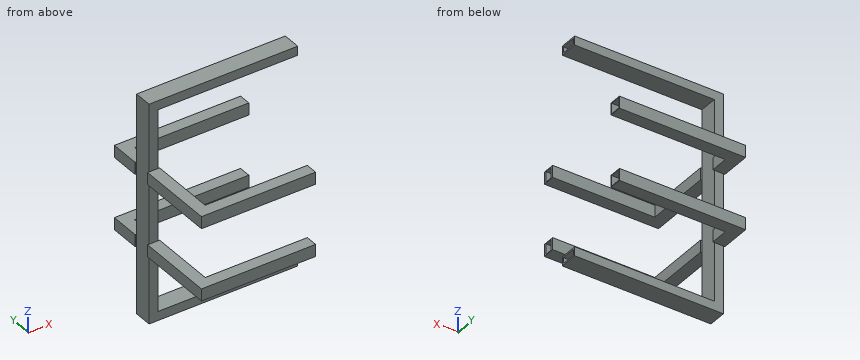
Autodesk Inventor part; units mm, degrees
ref_plane "Work Plane2" through (304.8, 0, 0) normal (1, 0, 0) x (0, 1, 0)
ref_plane "Work Plane3" through (0, 0, 50.8) normal (0, 0, 1) x (1, 0, 0)
ref_plane "Work Plane5" through (0, 0, 76.2) normal (0, 0, 1) x (1, 0, 0)
sketch "Sketch10" plane through (0, 0, 0) normal (0, 1, 0) x (-1, 0, 0)
  line L0 (0, 0) -> (0, 222.25)
  line L1 (0, 222.25) -> (-304.8, 222.25)
  line L2 (0, 0) -> (-304.8, 0) construction
  line L3 (0, 0) -> (0, -222.25)
  line L4 (0, -222.25) -> (-304.8, -222.25)
  dimension "d31" = 222.25
  dimension "d32" = 304.8
ref_plane "Work Plane2" through (304.8, 0, 0) normal (1, 0, 0) x (0, 1, 0)
sketch "Sketch11" plane through (304.8, 0, 0) normal (1, 0, 0) x (0, 1, 0)
  line L0 (-19.05, 231.775) -> (-19.05, 212.725)
  line L1 (-19.05, 212.725) -> (19.05, 212.725)
  line L2 (19.05, 212.725) -> (19.05, 231.775)
  line L3 (19.05, 231.775) -> (-19.05, 231.775)
  line L4 (-19.05, 231.775) -> (19.05, 212.725) construction
  line L5 (-19.05, 212.725) -> (19.05, 231.775) construction
  line L6 (-15.875, 228.6) -> (-15.875, 215.9)
  line L7 (-15.875, 215.9) -> (15.875, 215.9)
  line L8 (15.875, 215.9) -> (15.875, 228.6)
  line L9 (15.875, 228.6) -> (-15.875, 228.6)
  line L10 (-15.875, 228.6) -> (15.875, 215.9) construction
  line L11 (-15.875, 215.9) -> (15.875, 228.6) construction
  point P0 (0, 0)
  point P1 (0, 222.25)
  dimension "d34" = 222.25
  dimension "d35" = 19.05
  dimension "d36" = 38.1
  dimension "d37" = 3.175
  dimension "d38" = 3.175
sweep "Sweep5" add profiles "Sketch11" path "Sketch10"
sketch "Sketch12" plane through (304.8, 19.05, 231.775) normal (0, 1, 0) x (1, 0, 0)
  line L0 (-304.8, 231.775) -> (-304.8, 0) construction
  line L1 (0, 0) -> (-314.325, 0) construction
  line L2 (-317.5, 142.875) -> (-292.1, 142.875)
  line L3 (-292.1, 142.875) -> (-292.1, 168.275)
  line L4 (-292.1, 168.275) -> (-317.5, 168.275)
  line L5 (-317.5, 168.275) -> (-317.5, 142.875)
  line L6 (-317.5, 142.875) -> (-292.1, 168.275) construction
  line L7 (-292.1, 142.875) -> (-317.5, 168.275) construction
  line L8 (-298.45, 15.875) -> (-298.45, 447.675)
  line L9 (-315.9125, 144.4625) -> (-293.6875, 144.4625)
  line L10 (-293.6875, 144.4625) -> (-293.6875, 166.6875)
  line L11 (-293.6875, 166.6875) -> (-315.9125, 166.6875)
  line L12 (-315.9125, 166.6875) -> (-315.9125, 144.4625)
  line L13 (-315.9125, 144.4625) -> (-293.6875, 166.6875) construction
  line L14 (-293.6875, 144.4625) -> (-315.9125, 166.6875) construction
  point P0 (-304.8, 155.575)
  dimension "d41" = 25.4
  dimension "d42" = 25.4
  dimension "d43" = 76.2
  dimension "d44" = 1.5875
  dimension "d45" = 1.5875
ref_plane "Work Plane3" through (0, 0, 50.8) normal (0, 0, 1) x (1, 0, 0)
sketch "Sketch13" plane through (0, 0, 50.8) normal (0, 0, 1) x (1, 0, 0)
  line L0 (304.8, 19.05) -> (-9.525, 19.05)
  line L1 (0, 19.05) -> (0, 69.85)
  line L2 (0, 69.85) -> (254, 69.85)
  point P0 (0, 0)
  dimension "d47" = 254
  dimension "d48" = 50.8
sweep "Sweep6" add profiles "Sketch12" path "Sketch13" path curves L1 L2 contours L5 L4 L8 L11 L12 L9 L2 | L8 L9 L10 L11 L4 L3 L2
mirror "Mirror2" about plane through (0, 0, 0) normal (0, 0, 1) of "Sweep6"
sketch "Sketch14" plane through (304.8, -19.05, 212.725) normal (0, -1, 0) x (1, 0, 0)
  line L0 (-304.8, -212.725) -> (-304.8, 15.875) construction
  line L1 (0, 15.875) -> (-311.15, 15.875) construction
  line L2 (-317.5, -123.825) -> (-317.5, -149.225)
  line L3 (-317.5, -149.225) -> (-292.1, -149.225)
  line L4 (-292.1, -149.225) -> (-292.1, -123.825)
  line L5 (-292.1, -123.825) -> (-317.5, -123.825)
  line L6 (-317.5, -123.825) -> (-292.1, -149.225) construction
  line L7 (-317.5, -149.225) -> (-292.1, -123.825) construction
  line L8 (-312.7375, -125.4125) -> (-312.7375, -147.6375)
  line L9 (-312.7375, -147.6375) -> (-296.8625, -147.6375)
  line L10 (-296.8625, -147.6375) -> (-296.8625, -125.4125)
  line L11 (-296.8625, -125.4125) -> (-312.7375, -125.4125)
  line L12 (-312.7375, -125.4125) -> (-296.8625, -147.6375) construction
  line L13 (-312.7375, -147.6375) -> (-296.8625, -125.4125) construction
  line L14 (-314.325, 19.05) -> (-314.325, -444.5)
  point P0 (-304.8, -136.525)
  dimension "d52" = 76.2
  dimension "d53" = 25.4
  dimension "d54" = 25.4
  dimension "d55" = 1.5875
  dimension "d56" = 1.5875
ref_plane "Work Plane5" through (0, 0, 76.2) normal (0, 0, 1) x (1, 0, 0)
sketch "Sketch15" plane through (0, 0, 76.2) normal (0, 0, 1) x (1, 0, 0)
  line L0 (-9.525, -19.05) -> (304.8, -19.05)
  line L1 (0, -19.05) -> (0, -171.45)
  line L2 (0, -171.45) -> (228.6, -171.45)
  point P0 (0, 0)
  dimension "d58" = 228.6
  dimension "d59" = 152.4
sweep "Sweep7" add profiles "Sketch14" path "Sketch15" path curves L1 L2
mirror "Mirror5" about plane through (0, 0, 0) normal (0, 0, 1) of "Sweep7"
ref_plane "Work Plane6" through (152.4, 0, 0) normal (1, 0, 0) x (0, 1, 0)
equation "\"d31\" = halfOfWidth"
equation "\"d32\" = length"
equation "\"d35\" = largeTubingWidth"
equation "\"d36\" = largeTubingHeight"
equation "\"d37\" = largeTubeThickness"
equation "\"d38\" = largeTubeThickness"
equation "\"d41\" = smallSupportTubeWidth"
equation "\"d42\" = smallSupportTubeWidth"
equation "\"d44\" = smallSupportTubeThickness"
equation "\"d45\" = smallSupportTubeThickness"
equation "\"d47\" = topSupportTubeExtension"
equation "\"d48\" = smallSupportTubeLength"
equation "\"d53\" = smallSupportTubeWidth"
equation "\"d54\" = smallSupportTubeHeight"
equation "\"d55\" = smallSupportTubeThickness"
equation "\"d56\" = smallSupportTubeThickness"
equation "\"d58\" = bottomSupportTubeExtension"
equation "\"halfOfWidth\" = 0.5 * width"
equation "\"length\" = 304.8"
equation "\"height\" = 241.3"
equation "\"largeTubingWidth\" = 19.05"
equation "\"largeTubingHeight\" = 38.1"
equation "\"largeTubeThickness\" = 3.175"
equation "\"d33\" = length"
equation "\"width\" = 444.5"
equation "\"smallSupportTubeWidth\" = 25.4"
equation "\"smallSupportTubeHeight\" = 25.4"
equation "\"smallSupportTubeThickness\" = 1.5875"
equation "\"distaceToMiddleSmallSupportTube\" = 76.2"
equation "\"smallSupportTubeLength\" = 50.8"
equation "\"d46\" = smallSupportTubeLength"
equation "\"d57\" = distaceToMiddleSmallSupportTube"
equation "\"distanceOriginToPlaneForSupportTubes\" = 152.4"
equation "\"d62\" = distanceOriginToPlaneForSupportTubes"
properties part number "ShooterFrameV03"
The listing builds one solid part. Answer for the finished solid, in the listing's coordinates (mm). Give positions to 0.01 mm unless a question says otherwise; leave off trailing zeros. Order: outer loops, then holes, each group sorted by start corner. A loop starts at its lowest first (then second) coordinate and runs counter-clockwise, first axis right, second up. Notation, with made-up numbers: M 1.25,74.25 L 42.25,74.25 A4 cw 42.25,78.25 Z; hole C -5.5,12.5 d11. An arc over 180 degrees is marked long. Put each result on its own line as item: value. Start each with the question number.
Item 1: The part is cut by section A-A, the plane y = 41. Determine the outline of the cut face in (x, z), and give its area (3 significant figures).
Item 2: The part is cut by section D-D, the plane x = 67. State how many separate pieces and enclosed holes the cut face has, and give its area (3 significant figures).
Item 3: The part is cut by section B-B, the plane y = 8.5. Determine the outline of the cut face in (x, z) (3 decimals).
Item 4: Flat-ended cylindrical pins translate along their axes: P1, Ø9.5, axis at y = 4, z = 100, coming from the +X side (3 decimals); P2, Ø21, axis at x = 2.5, z = 25, coming from the +Y side; P3, Ø12, axis at x = 216, y = 52.5, coming from the -Z side. Find the tip coordinate at first contact, or state that the pin passes through.
Item 5: The part is cut by section C-C, the plane z = 139. Determine the outline of the cut face in (x, y) (3 decimals), and give its area (3 significant figures).
Item 6: Find the intervals of material crossed by line 1 along Y through (x, z) = (193, -81.5); line 2 along Z through (x, y) = (204, -1.5) (3 decimals); line 3 along Z through (x, y) = (30, 60), in increasing order.
Answer key:
1. outline: M -12.7,-88.9 L 12.7,-88.9 L 12.7,-63.5 L -12.7,-63.5 Z; M -12.7,63.5 L 12.7,63.5 L 12.7,88.9 L -12.7,88.9 Z; hole M -11.11,-87.31 L 11.11,-87.31 L 11.11,-65.09 L -11.11,-65.09 Z; hole M -11.11,65.09 L 11.11,65.09 L 11.11,87.31 L -11.11,87.31 Z
1. area: 302 mm²
2. separate pieces: 6
2. enclosed holes: 6
2. area: 1,530 mm²
3. outline: M -9.525,-231.775 L 304.8,-231.775 L 304.8,-228.6 L -6.35,-228.6 L -6.35,228.6 L 304.8,228.6 L 304.8,231.775 L -9.525,231.775 Z; M 6.35,-215.9 L 304.8,-215.9 L 304.8,-212.725 L 9.525,-212.725 L 9.525,212.725 L 304.8,212.725 L 304.8,215.9 L 6.35,215.9 Z
4. P1: stops at x = 9.525
4. P2: stops at y = 19.05
4. P3: stops at z = -88.9
5. outline: M -9.525,-19.05 L 9.525,-19.05 L 9.525,19.05 L -9.525,19.05 Z; hole M -6.35,-15.875 L 6.35,-15.875 L 6.35,15.875 L -6.35,15.875 Z
5. area: 323 mm²
6. line 1: y = -184.15 to -179.39, -163.51 to -158.75, 57.15 to 58.74, 80.96 to 82.55
6. line 2: z = -231.775 to -228.6, -215.9 to -212.725, 212.725 to 215.9, 228.6 to 231.775
6. line 3: z = -88.9 to -87.31, -65.09 to -63.5, 63.5 to 65.09, 87.31 to 88.9
